Geometry: see drawing. Coordinates: mm, zero at the bounding-box minimum. A direction names the side the tool comes from. Coordinates: 2 decimals unless noted, no trailing zeros. Loops run counter-clockwise (first coordinate to the right, second up) from the corner with the lowest first, then second, coordinate; pieces in that order, holes last. Notation, with made-up numbers: (-35, -34.5) -> (-26, -34.5) arc R13 ccw to (-26, -15.5) -> close; hole circle Ø6 at (12, 32). An arc over 180 degrees is marked (long way). Answer as a JSON object with one key per item and string values.
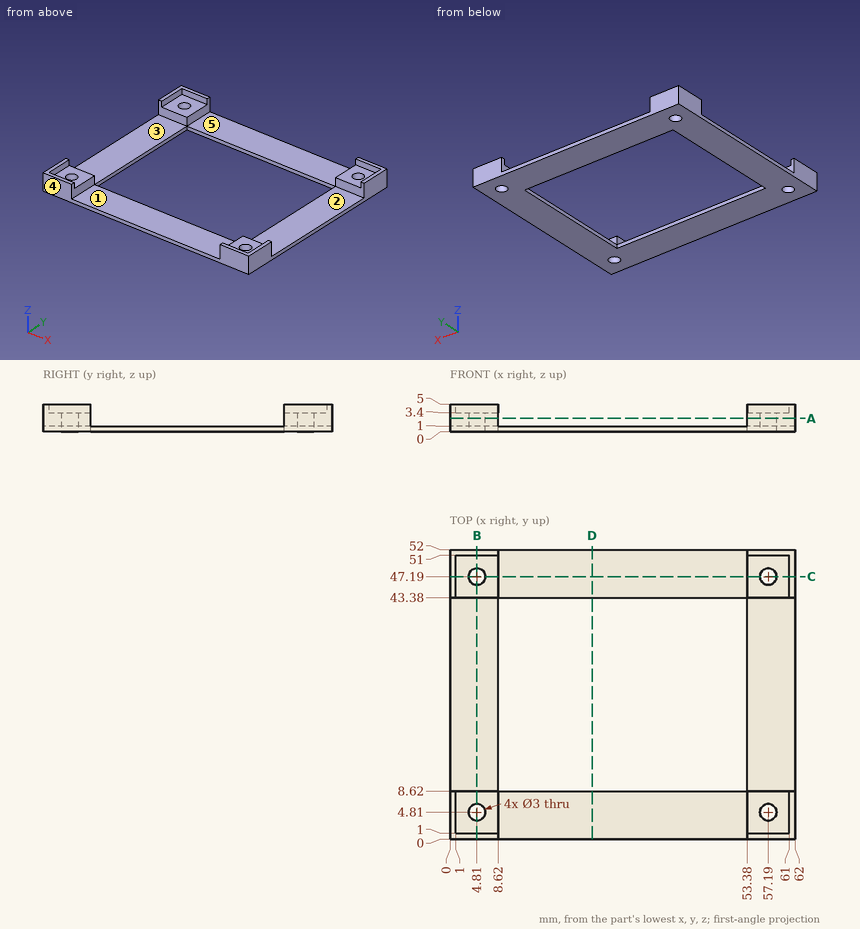
1. Pin query (flat end, axial travel): P1, Ø3, axis at y = 25, z = 4, coming from the +X side; P2, Ø4, axis at x = 57.19, y = 4.81, coming from the +Z side. Return the tip coordinate at first contact, or that it passes through.
Reply:
{"P1": "passes through", "P2": "stops at z = 3.4"}
2. Section query C-C (y = 47.19). Return loops of the section in (x, z).
Reply:
{"outline": "(0, 0) -> (3.31, 0) -> (3.31, 3.4) -> (1, 3.4) -> (1, 5) -> (0, 5) -> close; (6.31, 0) -> (55.69, 0) -> (55.69, 3.4) -> (53.38, 3.4) -> (53.38, 1) -> (8.62, 1) -> (8.62, 3.4) -> (6.31, 3.4) -> close; (58.69, 0) -> (62, 0) -> (62, 5) -> (61, 5) -> (61, 3.4) -> (58.69, 3.4) -> close"}
3. Section query B-B (x = 4.81). Return loops of the section in (y, z), plus the area to 3 significant figures.
Reply:
{"outline": "(0, 0) -> (3.31, 0) -> (3.31, 3.4) -> (1, 3.4) -> (1, 5) -> (0, 5) -> close; (6.31, 0) -> (45.69, 0) -> (45.69, 3.4) -> (43.38, 3.4) -> (43.38, 1) -> (8.62, 1) -> (8.62, 3.4) -> (6.31, 3.4) -> close; (48.69, 0) -> (52, 0) -> (52, 5) -> (51, 5) -> (51, 3.4) -> (48.69, 3.4) -> close", "area": "76.2 mm2"}
4. Section query A-A (z = 2.4). Return loops of the section in (x, y), plus the area to 3 significant figures.
Reply:
{"outline": "(0, 0) -> (8.62, 0) -> (8.62, 8.62) -> (0, 8.62) -> close; (0, 43.38) -> (8.62, 43.38) -> (8.62, 52) -> (0, 52) -> close; (53.38, 0) -> (62, 0) -> (62, 8.62) -> (53.38, 8.62) -> close; (53.38, 43.38) -> (62, 43.38) -> (62, 52) -> (53.38, 52) -> close; hole circle Ø3 at (4.81, 4.81); hole circle Ø3 at (4.81, 47.19); hole circle Ø3 at (57.19, 4.81); hole circle Ø3 at (57.19, 47.19)", "area": "269 mm2"}
5. Mould query, pull axis X, two halves, no side actions, for the marked faces 1 and 2. Classes: pulls with the +X half, pulls with the -X half, needs draft (parallel to the pull), parting line crosses it, or undercut.
Reply:
{"face 1": "undercut", "face 2": "needs draft"}
6. Line query: line 1 along Y through (x, z) = (4.81, 2.05); line 2 along X through (y, z) = (4.81, 1.25); line 3 along X through (y, z) = (47.19, 0.95). Output: solid intervals per line, ascending.
Reply:
{"line 1": "y = 0 to 3.31, 6.31 to 8.62, 43.38 to 45.69, 48.69 to 52", "line 2": "x = 0 to 3.31, 6.31 to 8.62, 53.38 to 55.69, 58.69 to 62", "line 3": "x = 0 to 3.31, 6.31 to 55.69, 58.69 to 62"}
7. Section query D-D (x = 25.5). Return loops of the section in (y, z), plus the area to 3 significant figures.
Reply:
{"outline": "(0, 0) -> (8.62, 0) -> (8.62, 1) -> (0, 1) -> close; (43.38, 0) -> (52, 0) -> (52, 1) -> (43.38, 1) -> close", "area": "17.2 mm2"}
8. Access query for the marked faces 3, 4 and 5. Directions: +Z, -Z, +X, -X, +Y, -Y. A direction counts if a zero-diameter tool reaches every point of the face in a straight line with its end or side. Return the directions, or none.
Reply:
{"face 3": "+Z, +X, -X", "face 4": "+Z, -Z, +X, -X, -Y", "face 5": "+Z, +Y, -Y"}
